from build123d import *

# Parameters (mm, degrees)
EXTRUDE_THIN1_DEPTH = 1016
FILLET1_R           = 1.27


with BuildPart() as part:
    # Sketch1 → Extrude-Thin1 (new body)
    with BuildSketch(Plane.XY):
        with BuildLine():
            Line((0, 0), (-25.4, 0))
            ThreePointArc((-25.4, 0), (-26.266516, 2.861906), (-28.575, 4.7625))
            ThreePointArc((-28.575, 4.7625), (-30.883484, 6.663094), (-31.75, 9.525))
            Line((-31.75, 9.525), (-35.71875, 9.525))
            Line((-35.71875, 9.525), (-35.71875, 46.0375))
            Line((-35.71875, 46.0375), (-39.6875, 46.0375))
            Line((-39.6875, 46.0375), (-39.6875, 52.3875))
            ThreePointArc((-39.6875, 52.3875), (-49.260127, 56.036408), (-53.975, 65.131445))
            ThreePointArc((-53.975, 65.131445), (-58.111252, 73.680907), (-66.675, 77.7875))
            Line((-66.675, 77.7875), (-66.675, 101.6))
            Line((-66.675, 101.6), (-53.975, 101.6))
            Line((-53.975, 101.6), (-53.975, 100.33))
            Line((-53.975, 100.33), (-65.405, 100.33))
            Line((-65.405, 100.33), (-65.405, 78.882323))
            ThreePointArc((-65.405, 78.882323), (-56.817633, 74.169998), (-52.713255, 65.276013))
            ThreePointArc((-52.713255, 65.276013), (-47.930054, 56.572496), (-38.4175, 53.719154))
            Line((-38.4175, 53.719154), (-38.4175, 47.3075))
            Line((-38.4175, 47.3075), (-34.44875, 47.3075))
            Line((-34.44875, 47.3075), (-34.44875, 10.795))
            Line((-34.44875, 10.795), (-30.26681, 10.795))
            ThreePointArc((-30.26681, 10.795), (-30.139289, 7.933077), (-28.086538, 5.934808))
            ThreePointArc((-28.086538, 5.934808), (-25.590211, 4.079739), (-24.25668, 1.27))
            Line((-24.25668, 1.27), (0, 1.27))
            Line((0, 1.27), (0, 0))
        make_face()
    extrude(amount=-EXTRUDE_THIN1_DEPTH)

    # Fillet1
    fillet1_edges = [part.edges().sort_by_distance(p)[0] for p in [
        (-38.4175, 53.719154, -508),
        (-34.44875, 47.3075, -508),
        (-30.26681, 10.795, -508),
        (-25.4, 0, -508),
        (-35.71875, 9.525, -508),
        (-39.6875, 46.0375, -508),
        (-66.675, 77.7875, -508),
        (-66.675, 101.6, -508),
    ]]
    fillet(fillet1_edges, radius=FILLET1_R)


solid = part.part
Read the model definition and answer for the solid it produces. Units are mm, in the model's axes. A direction names the side the tool comes from. Give positions to 0.01 mm unless a question says otherwise; leave off trailing zeros. Loops run counter-clockwise (first coordinate to the right, second up) from the corner with the lowest first, then second, coordinate; pieces in that order, holes last. Notation, with made-up numbers: (38.5, -6.75) -> (84.5, -6.75) arc R25 ccw to (84.5, 31.25) -> close; hole circle Ø3 at (-33, -1.5). An arc over 180 degrees is marked (long way). Use a Markdown table: item, result.
Q1. Section C-C, the plane x = -9 is taken. Determine the outline of the cut face in (y, z), then the cut area to 3 significant figures.
Solved:
| item | result |
|---|---|
| outline | (0, -1016) -> (1.27, -1016) -> (1.27, 0) -> (0, 0) -> close |
| area | 1,290 mm^2 |
Q2. Determine the mould class of faces 1 (the face through (-12, 1.27, -501)), 2 (the face through (-38, 47, -1016)), 3 (the face through (-65.405, 90, -501)), 4 (the face through (-12, 0, -501)) for opening direction Y: pulls with the +Y half, pulls with the -Y half, needs draft (parallel to the pull), parting line crosses it, or undercut.
Solved:
| item | result |
|---|---|
| face 1 | pulls with the +Y half |
| face 2 | needs draft |
| face 3 | undercut |
| face 4 | pulls with the -Y half |
Q3. A tool of negligible diameter and unlimited length cuts with its end or side. For faces 5 (the face through (-35.719, 28, -501)), 6 (the face through (-38, 47, 0)), 7 (the face through (-34.449, 29, -501)), from which of +Z, -Z, +X, -X, +Y, -Y can it reach the whole face along a straight path? Write none if from no direction.
Solved:
| item | result |
|---|---|
| face 5 | +Z, -Z, -X, -Y |
| face 6 | +Z, +X, -X, +Y, -Y |
| face 7 | +Z, -Z, +X, +Y |
Q4. Section B-B, the plane y = 31 is taken. Determine the outline of the cut face in (x, z), then the cut area to 3 significant figures.
Solved:
| item | result |
|---|---|
| outline | (-35.72, -1016) -> (-34.45, -1016) -> (-34.45, 0) -> (-35.72, 0) -> close |
| area | 1,290 mm^2 |
Q5. Each of these flat-tipped pins is pushed along its axis until it touches: pin 1 (1 mm diameter, centred on y = 100.5, z = -554, fed in from +X) (3 decimals); pin 2 (4 mm diameter, centred on y = 49, z = -497, fed in from +X); pin 3 (7.5 mm diameter, centred on x = -6.5, z = -692, fed in from +Y). Where does it stop, or does it pass through?
Solved:
| item | result |
|---|---|
| pin 1 | stops at x = -53.975 |
| pin 2 | stops at x = -34.89 |
| pin 3 | stops at y = 1.27 |
Q6. Find the intervals of material crossed by line 1 along X through (y, z) = (14.5, -865); line 2 along Y through (x, z) = (-3.5, -228.5); line 3 along X through (y, z) = (49.5, -166.5), in increasing order.
Solved:
| item | result |
|---|---|
| line 1 | x = -35.72 to -34.45 |
| line 2 | y = 0 to 1.27 |
| line 3 | x = -39.69 to -38.42 |
